Could you check a few things on this drawing? It's one solid part, dimensions in mm from its lowest x, y, z. A direction names the side the tool comes from. Give positions to 0.01 mm unless a question says otherwise; leave off trailing zeros. Order: outer loops, then holes, each group sorted by start corner. A loop starts at its lowest first (then second) coordinate and runs counter-clockwise, first axis right, second up. Notation, with made-up numbers: (56, 52) -> (107, 52) arc R24 cw to (107, 88) -> close; hole circle Ø10 at (34.5, -33.75). An arc over 180 degrees is marked (long way). Write each question's results on one line, items separated by ' | '.
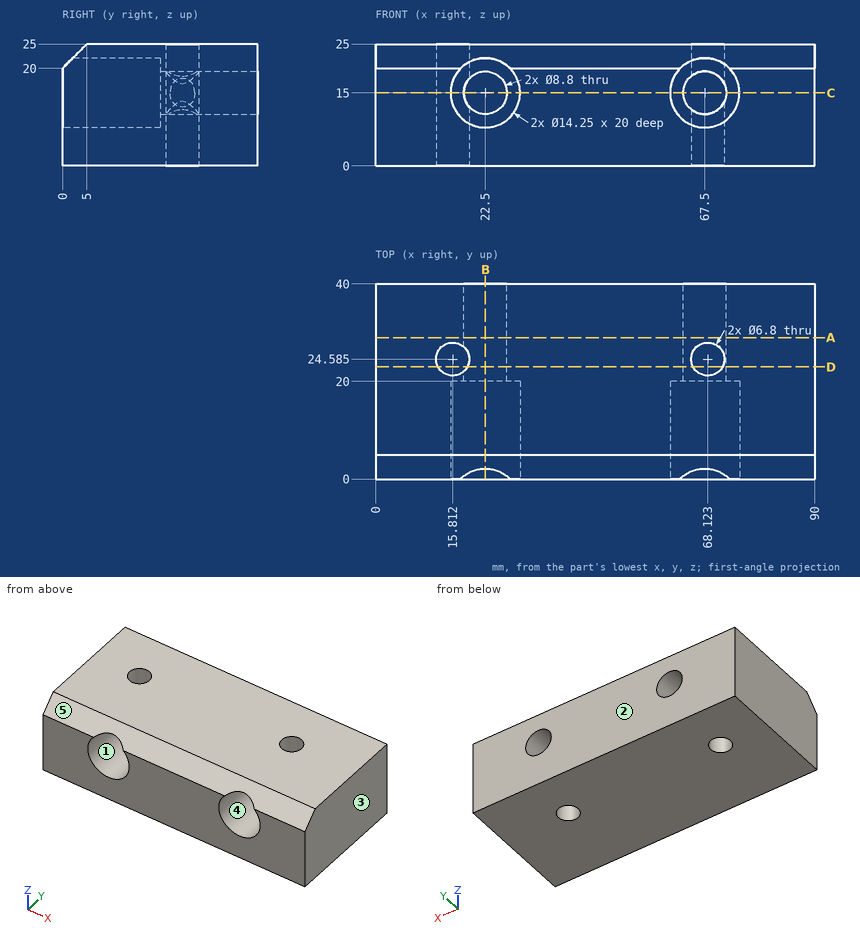
Q1. I'm going to push a flat-ended pin straight in: pin 1 Ø7 at (x, z) = (24, 13.5) entering from -Y. Where does the tip first touch, or does it pass through?
Here are the results:
pin 1: stops at y = 20
Q2. Suppose I cut it at A-A on y = 29. Please give me the cut outline in (x, z).
Here are the results:
outline: (0, 0) -> (90, 0) -> (90, 25) -> (0, 25) -> close; hole circle Ø8.8 at (22.5, 15); hole circle Ø8.8 at (67.5, 15)
Q3. For the marked faces 4 and 5, which set-ups out of +Z, -Z, +X, -X, +Y, -Y let a thin tool reach every point of the face, with its end or its side?
Here are the results:
face 4: -Y | face 5: +Z, +X, -X, -Y
Q4. Suppose I cut it at D-D on y = 23. Please give me the cut outline in (x, z) (1 decimal), and give its area (3 significant figures).
Here are the results:
outline: (0, 0) -> (12.8, 0) -> (12.8, 25) -> (0, 25) -> close; (18.8, 0) -> (65.1, 0) -> (65.1, 11.3) arc R4.4 cw to (65.1, 18.7) -> (65.1, 25) -> (18.8, 25) -> (18.8, 17.4) arc R4.4 cw (long way) to (18.8, 12.6) -> close; (71.1, 0) -> (90, 0) -> (90, 25) -> (71.1, 25) -> (71.1, 17.5) arc R4.4 cw to (71.1, 12.5) -> close | area: 1,880 mm²
Q5. Suppose I cut it at B-B on x = 22.5. Please give me the cut outline in (y, z) (1 decimal).
Here are the results:
outline: (0, 0) -> (40, 0) -> (40, 10.6) -> (20, 10.6) -> (20, 7.9) -> (0, 7.9) -> close; (2.1, 22.1) -> (20, 22.1) -> (20, 19.4) -> (40, 19.4) -> (40, 25) -> (5, 25) -> close
Q6. Thinking about a two-plate mould opening in X: for the marked faces 1, 2 and 3, which applies, +X half, -X half, draft (parallel to the pull), parting line (faces both ways), or undercut?
Here are the results:
face 1: undercut | face 2: draft | face 3: +X half
Q7. Suppose I cut it at C-C on z = 15. Please give me the cut outline in (x, y) (1 decimal).
Here are the results:
outline: (0, 0) -> (15.4, 0) -> (15.4, 20) -> (18.1, 20) -> (18.1, 22.1) arc R3.4 cw (long way) to (18.1, 27.1) -> (18.1, 40) -> (0, 40) -> close; (26.9, 20) -> (29.6, 20) -> (29.6, 0) -> (60.4, 0) -> (60.4, 20) -> (63.1, 20) -> (63.1, 40) -> (26.9, 40) -> close; (71.9, 20) -> (74.6, 20) -> (74.6, 0) -> (90, 0) -> (90, 40) -> (71.9, 40) -> close
Q8. I need wall thicknesses on line 1 along Y through (x, z) = (68, 6.5); line 2 along X through (y, z) = (33.5, 16.75); line 3 along X through (y, z) = (24, 5.25). Which ranges of each line are inside material? Lowest first, please.
Here are the results:
line 1: y = 0 to 21.19, 27.98 to 40 | line 2: x = 0 to 18.46, 26.54 to 63.46, 71.54 to 90 | line 3: x = 0 to 12.46, 19.16 to 64.77, 71.47 to 90
